Read the model definition and answer for the solid it produces. Units are mm, in the model's axes. A direction names the side the tool comes from. Give positions to 0.01 mm unless a question says otherwise; leave off trailing zeros. Order: outer loops, then holes, each group sorted by start corner. A loop starts at its lowest first (then second) coordinate and runs counter-clockwise, first axis right, second up. Notation, with made-up numbers: (33, 70) -> (43, 70) arc R25 ccw to (43, 97) -> close; hole circle Ø5 at (18.25, 14). An arc over 180 degrees is marked (long way). Use one line per item in the form item = value.
```python
from build123d import *

# Parameters (mm, degrees)
F1_DEPTH = 4
F2_SIZE  = 2.3
F3_SIZE  = 1.99999


# Not quite as in the source:
# - a fillet or chamfer is up to 0.001 mm smaller than in the source, because OpenCascade refuses the exact size


with BuildPart() as f1:
    # F0 (on Top) → F1 (new body)
    with BuildSketch(Plane.XY):
        Polygon((-75.4356830697, -28.6679565907), (-75.4356830697, -30), (44.5643169303, -30), (44.5643169303, 0), (37.0643169303, 0), (37.0643169303, -10), (37.0643169303, -15.06), (22.0643169303, -15.06), (22.0643169303, -10), (22.0643169303, 0), (7.0643169303, 0), (7.0643169303, -10), (7.0643169303, -15.06), (-7.9356830697, -15.06), (-7.9356830697, -10), (-7.9491234598, 0), (-22.9491234598, 0), (-22.9491234598, -10), (-22.9491234598, -15.06), (-37.9491234598, -15.06), (-37.9491234598, -10), (-37.9491234598, 0), (-52.9491234598, 0), (-52.9491234598, -10), (-52.9229563225, -15.06), (-67.9233574687, -15.06), (-67.9491234598, -10.077570565), (-67.9491234598, -0.077570565), (-75.4356830697, 0), (-75.4356830697, -15.06), align=None)
    extrude(amount=F1_DEPTH)

    # F2
    f2_edges = [f1.edges().sort_by_distance(p)[0] for p in [
        (-75.435683, 0, 2),
    ]]
    chamfer(f2_edges, length=F2_SIZE)

    # F3 (size 2 in the source; OpenCascade refuses exactly that, so slightly less here)
    f3_edges = [f1.edges().sort_by_distance(p)[0] for p in [
        (-75.435683, -16.15, 0),
        (-75.435683, -16.15, 4),
    ]]
    chamfer(f3_edges, length=F3_SIZE)


solid = f1.part
```
Item 1: The part is cut by section C-C on x = -5.5. Give the vertices of the cut face in (y, z).
Checks:
outline = (-30, 0) -> (-15.06, 0) -> (-15.06, 4) -> (-30, 4) -> close
Item 2: Straight lines are drawn through the part: L1, parallel to X at y = -10, z = 1.45; L2, parallel to X at y = -10, z = 1.25; L3, parallel to Y at x = -56, z = 1.65. For each, find the intervals that lie inside material, in ascending order. Write a range as from..to.
Checks:
L1 = -74.89..-67.95, -52.95..-37.95, -22.95..-7.94, 7.06..22.06, 37.06..44.56
L2 = -74.69..-67.95, -52.95..-37.95, -22.95..-7.94, 7.06..22.06, 37.06..44.56
L3 = -30..-15.06
Item 3: The part is cut by section B-B on z = 2.7. Give the vertices of the cut face in (x, y).
Checks:
outline = (-74.74, -30) -> (44.56, -30) -> (44.56, 0) -> (37.06, 0) -> (37.06, -15.06) -> (22.06, -15.06) -> (22.06, 0) -> (7.06, 0) -> (7.06, -15.06) -> (-7.94, -15.06) -> (-7.94, -10) -> (-7.95, 0) -> (-22.95, 0) -> (-22.95, -15.06) -> (-37.95, -15.06) -> (-37.95, 0) -> (-52.95, 0) -> (-52.95, -10) -> (-52.92, -15.06) -> (-67.92, -15.06) -> (-67.95, -10.08) -> (-67.95, -0.08) -> (-73.14, -0.02) -> (-74.74, -1.61) -> close
Item 4: The part is cut by section A-A on y = -9. State how many separate pieces and enclosed holes the cut face has, and give its area (3 significant figures).
Checks:
separate_pieces = 5
enclosed_holes = 0
area = 236 mm²
Item 5: Which of the six approach directions +Z, -Z, +X, -X, +Y, -Y give full straight-line access (tool end or side, diameter ignored) to faces 1 (the flat face through (-67.949, -5, 2)), 2 (the flat face through (15, 0, 2))?
Checks:
face_1 = +Z, -Z, +Y
face_2 = +Z, -Z, +X, -X, +Y
